For this review, take the finished solid that the model builds, in its own axes (mm). A direction names the side the tool comes from. Coordinates: 2 decimals unless noted, no trailing zeros. Write each loop counter-clockwise with the first axis right and the second up, starting at its lowest first coordinate (ties: lowest second). Pieces come first, ordered by that corner, then holes.
1) For faces 1 (the face through (1, -2, 115)), 2 (the face through (2.285, 3.584, 4.465)), list the 3-axis set-ups (+Z, -Z, +X, -X, +Y, -Y) from which the entire face can be reached by the end or side of a thin tool; tool diameter is ignored.
2) To check wall thickness, follow line 1 along Y through (x, z) = (0, 114); line 2 along X through (y, z) = (1.5, 34.5); line 3 along Z through (x, y) = (2.75, -3). State the ranges of each line that lie inside material, in increasing order.
3) Insertion check: P1, Ø2, axis at x = -2.5, z = 45.5, coming from the +Y side; P2, Ø1, axis at y = -1, z = 53, coming from the -X side. Each pin has a flat end and moves straight along its axis. Give the tip position at first contact, or say it passes through.
4) We need section C-C on z = 67.5. Write out the cut boundary in (x, y).
5) We need section A-A on y = 0. Write out the cut boundary in (x, z), then the cut area to 3 significant figures.
from build123d import *

# Parameters (mm, degrees)
M5_START                                       = 7
SKETCH1_R                                      = 2.5
M5_MOUNTING_BOLT_SHANK_AND_REDUCED_THREA_DEPTH = 108
M5_START_2                                     = 115
SKETCH2_R                                      = 2.02
M5_TAP_ENGAGEMENT_DEPTH                        = 7
SOCKET_START                                   = 2
SKETCH3_R                                      = 4.25
SOCKET_CAP_HEAD_DEPTH                          = 5


with BuildPart() as part:
    # Sketch1 → M5 mounting bolt shank and reduced thread representation (new body)
    with BuildSketch(Plane.XY.offset(M5_START)):
        Circle(SKETCH1_R)
    extrude(amount=M5_MOUNTING_BOLT_SHANK_AND_REDUCED_THREA_DEPTH)

    # Sketch2 → M5 tap engagement (add)
    with BuildSketch(Plane.XY.offset(M5_START_2)):
        Circle(SKETCH2_R)
    extrude(amount=M5_TAP_ENGAGEMENT_DEPTH)

    # Sketch3 → Socket cap head (add)
    with BuildSketch(Plane.XY.offset(SOCKET_START)):
        Circle(SKETCH3_R)
    extrude(amount=SOCKET_CAP_HEAD_DEPTH)


solid = part.part
Result:
1. face 1: +Z
1. face 2: +Z, -Z
2. line 1: y = -2.5 to 2.5
2. line 2: x = -2 to 2
2. line 3: z = 2 to 7
3. P1: stops at y = 2
3. P2: stops at x = -2.45
4. outline: circle Ø5 at (0, 0)
5. outline: (-4.25, 2) - (4.25, 2) - (4.25, 7) - (2.5, 7) - (2.5, 115) - (2.02, 115) - (2.02, 122) - (-2.02, 122) - (-2.02, 115) - (-2.5, 115) - (-2.5, 7) - (-4.25, 7) - close
5. area: 611 mm2
